Can you work these out from the model? Positions are in its coordinate system, mm. A direction names the side the tool comes from. Round coordinates to 2 decimals unless told otherwise and drop trailing zeros. Order: outer loops, then holes, each group sorted by start corner. A loop starts at its lowest first (then second) coordinate and runs counter-clockwise, first axis right, second up.
Q1. If we section it at B-B (x = -10.5): Please give me the cut outline in (y, z), plus the area to 3 significant figures.
Q2. For faces 5 (the face through (0, 25.9, 15)), 6 (the face through (0, 25, 16)), which set-ups out of +Z, -Z, +X, -X, +Y, -Y let a thin tool reach every point of the face, with its end or its side?
Q3. We'd pull the mould along Y, two halves only. Please class faces 1 (the face through (0, 0, 0)), 2 (the face through (0.35, 25.329, -0.358)), 3 (the face through (-25, 11.6, -0.3)), 4 (the face through (-0.35, -25.329, -0.358)): pulls with the +Y half, pulls with the -Y half, needs draft (parallel to the pull), parting line crosses it, or undercut.
Q4. If we section it at A-A (z = 22): Please give me the cut outline in (x, y).
Q5. If I drill on line 1 (Y direction, x = -8.5, z = 17); line 2 (Z direction, x = -16, y = 12.5), over which ranges is the centre line in solid material (lowest first)?
Q6. If we section it at C-C (y = 7.5): Please give me the cut outline in (x, z).
Q7. Will this pin go through, and if not, where does the flat tip stop? P1, Ø24, axis at x = -11, y = -8.5, coming from the +Z side.
from build123d import *

# Parameters (mm, degrees)
SKETCH1_W                    = 50
SKETCH1_H                    = 50
BASE_FLANGE1_DEPTH           = 0.9
EDGE_FLANGE1_STRIP_W         = 5.6
EDGE_FLANGE1_STRIP_H         = 0.9
EDGE_FLANGE1_STRIP_CUT_DEPTH = 50
EDGE_FLANGE1_DEPTH           = 50
EDGE_FLANGE2_STRIP_W         = 5.6
EDGE_FLANGE2_STRIP_H         = 0.9
EDGE_FLANGE2_STRIP_CUT_DEPTH = 50
EDGE_FLANGE2_DEPTH           = 50


# Sheet-metal steps are written as plain solids
with BuildPart() as part:
    # Sketch1 → Base-Flange1 (new body)
    with BuildSketch(Plane.XY):
        Rectangle(SKETCH1_W, SKETCH1_H)
    extrude(amount=-BASE_FLANGE1_DEPTH)

    # Edge-Flange1 strip (across the edge) → Edge-Flange1 strip cut (cut)
    with BuildSketch(Plane(origin=(25, 25, 0), x_dir=(0, -1, 0), z_dir=(-1, 0, 0))):
        with Locations((-1.8, -0.45)):
            Rectangle(EDGE_FLANGE1_STRIP_W, EDGE_FLANGE1_STRIP_H)
    extrude(amount=EDGE_FLANGE1_STRIP_CUT_DEPTH, mode=Mode.SUBTRACT)

    # Edge-Flange1 section (across the edge) → Edge-Flange1 (add)
    with BuildSketch(Plane(origin=(25, 25, 0), x_dir=(0, -1, 0), z_dir=(-1, 0, 0))):
        with BuildLine():
            Line((-0.9, 1), (-0.9, 30))
            Line((-0.9, 30), (0, 30))
            Line((0, 30), (0, 1))
            ThreePointArc((0, 1), (0.292893219, 0.292893219), (1, 0))
            Line((1, 0), (1, -0.9))
            ThreePointArc((1, -0.9), (-0.343502884, -0.343502884), (-0.9, 1))
        make_face()
    extrude(amount=EDGE_FLANGE1_DEPTH)

    # Edge-Flange2 strip (across the edge) → Edge-Flange2 strip cut (cut)
    with BuildSketch(Plane(origin=(-25, -25, 0), x_dir=(0, 1, 0), z_dir=(1, 0, 0))):
        with Locations((-1.8, -0.45)):
            Rectangle(EDGE_FLANGE2_STRIP_W, EDGE_FLANGE2_STRIP_H)
    extrude(amount=EDGE_FLANGE2_STRIP_CUT_DEPTH, mode=Mode.SUBTRACT)

    # Edge-Flange2 section (across the edge) → Edge-Flange2 (add)
    with BuildSketch(Plane(origin=(-25, -25, 0), x_dir=(0, 1, 0), z_dir=(1, 0, 0))):
        with BuildLine():
            Line((-0.9, 1), (-0.9, 30))
            Line((-0.9, 30), (0, 30))
            Line((0, 30), (0, 1))
            ThreePointArc((0, 1), (0.292893219, 0.292893219), (1, 0))
            Line((1, 0), (1, -0.9))
            ThreePointArc((1, -0.9), (-0.343502884, -0.343502884), (-0.9, 1))
        make_face()
    extrude(amount=EDGE_FLANGE2_DEPTH)


solid = part.part
Solution:
1. outline: (-25.9, 1) arc R1.9 ccw to (-24, -0.9) - (24, -0.9) arc R1.9 ccw to (25.9, 1) - (25.9, 30) - (25, 30) - (25, 1) arc R1 cw to (24, 0) - (-24, 0) arc R1 cw to (-25, 1) - (-25, 30) - (-25.9, 30) - close
1. area: 99.5 mm2
2. face 5: +Z, -Z, +X, -X, +Y
2. face 6: +Z, +X, -X
3. face 1: undercut
3. face 2: pulls with the +Y half
3. face 3: needs draft
3. face 4: pulls with the -Y half
4. outline: (-25, -25.9) - (25, -25.9) - (25, -25) - (-25, -25) - close; (-25, 25) - (25, 25) - (25, 25.9) - (-25, 25.9) - close
5. line 1: y = -25.9 to -25, 25 to 25.9
5. line 2: z = -0.9 to 0
6. outline: (-25, -0.9) - (25, -0.9) - (25, 0) - (-25, 0) - close
7. P1: stops at z = 0
